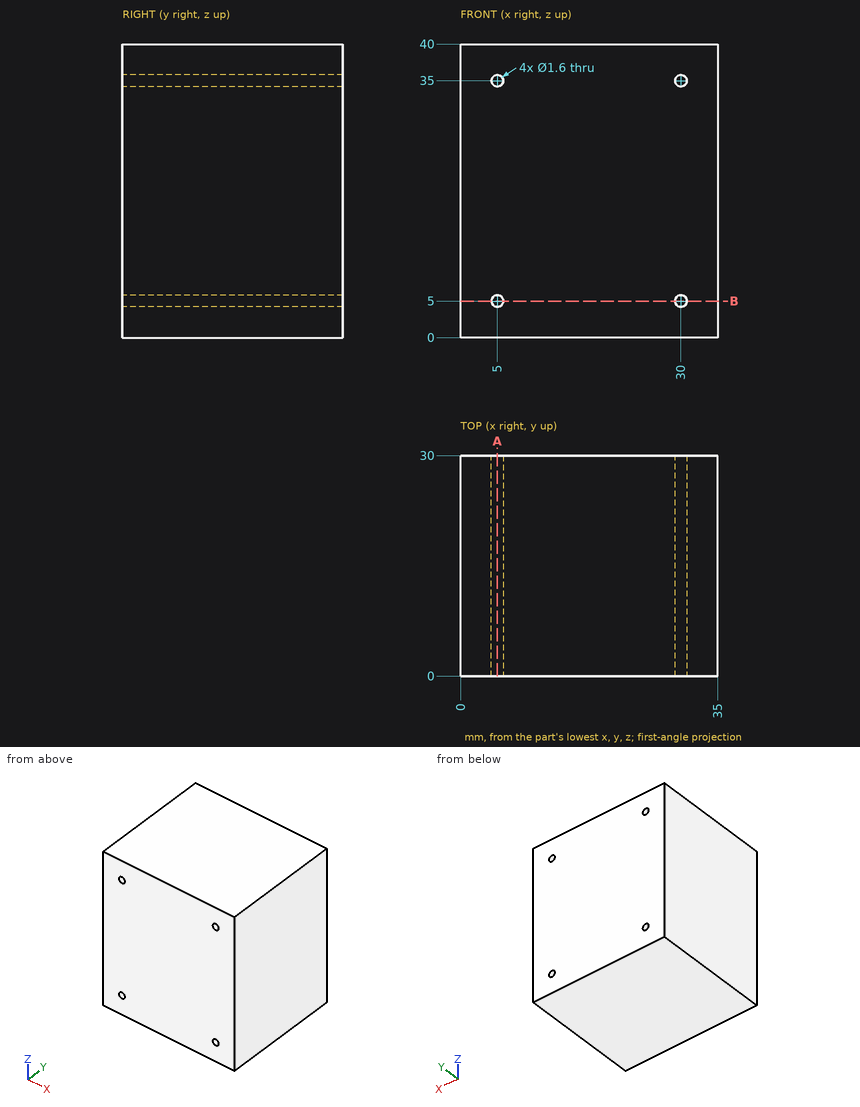
Job drawing, mm, ordinate dimensions from the low corner. One solid piece. Coordinates: 2 decimals unless noted, no trailing zeros. Write each loop counter-clockwise with the first axis right and the second up, starting at its lowest first coordinate (ties: lowest second). Pieces come first, ordered by that corner, then holes. Notation, with made-up numbers: (-36, 25.25) - (-3, 25.25) arc R22 ccw to (-3, 33.25) - close; hole circle Ø11 at (8.5, 80.25). An arc over 180 degrees is marked (long way). Use a Markdown table: item, result. Add a question column.
Item 1: Drill centre lines: L1, parallel to Z at x = 30, y = 15; L2, parallel to X at y = 19.25, z = 35; L3, parallel to Z at x = 5.5, y = 16.25. Where is each one in solid material? Low to high. Write a range as from..to.
Item 2: Flat gauge pins, fed straight in: pin 1 (3 mm diameter, centred on x = 25.5, y = 17.5, fed in from -Z); pin 2 (1.4 mm diameter, centred on x = 30, z = 35, fed in from -Y). Where does each tip first touch, or does it go through?
Item 3: Band-saw the part on B-B, the plane z = 5. Give the cut face in (x, y).
Item 4: Band-saw the part on A-A, the plane x = 5. Give the cut face in (y, z).
Numbers:
| question | item | result |
|---|---|---|
| 1 | L1 | 0..4.2, 5.8..34.2, 35.8..40 |
| 1 | L2 | 0..4.2, 5.8..29.2, 30.8..35 |
| 1 | L3 | 0..4.38, 5.62..34.38, 35.62..40 |
| 2 | pin 1 | z = 0 |
| 2 | pin 2 | through |
| 3 | outline | (0, 0) - (4.2, 0) - (4.2, 30) - (0, 30) - close; (5.8, 0) - (29.2, 0) - (29.2, 30) - (5.8, 30) - close; (30.8, 0) - (35, 0) - (35, 30) - (30.8, 30) - close |
| 4 | outline | (0, 0) - (30, 0) - (30, 4.2) - (0, 4.2) - close; (0, 5.8) - (30, 5.8) - (30, 34.2) - (0, 34.2) - close; (0, 35.8) - (30, 35.8) - (30, 40) - (0, 40) - close |
